Verification items for this drawing (mm, ordinates from the low corner). Round coordinates to 2 decimals unless told otherwise and drop trailing zeros. Order: outer loops, then holes, each group sorted by start corner. A loop starts at its lowest first (then second) coordinate and runs counter-clockwise, first axis right, second up. Notation, with made-up numbers: M 3,22 L 21,22 A6 cw 21,30 Z; hole C 21,68 d6. An arc over 180 degrees is marked long. Use CSV: the item, a comma, the result in double quotes. Start each with the question number.
Q1. Sectioned sample at A-A (z = 11.75). Enter the section's corners in (x, y), and give its area (3 significant figures).
Q2. Gauge pin test, flat ends, axial feed: pin 1 Ø2 at (y, z) = (49, 12.5) entering from -X; pin 2 Ø1.2 at (x, z) = (91.5, 12) entering from -Y; pin 3 Ø2 at (y, z) = (42.5, 12.5) entering from +X. Record the tip position at first contact, or that the pin passes through.
Q3. Sectioned sample at B-B (y = 52.5). Enter the section's corners in (x, z), and give its area (3 significant figures).
Q4. Mould release check, pull along Y, two halves, no side actions. Record for the marked faces 1 and 2: +Y half, -Y half, draft (parallel to the pull), parting line (faces both ways), or undercut.
Q5. Scan lines: line 1 (X direction, y = 70, z = 12.5); line 2 (Y direction, x = 36, z = 12.75); line 3 (Z direction, x = 92, y = 71). Record each from-to range of solid material in increasing order.
Q6. Sectioned sample at C-C (x = 27). Enter the section's corners in (y, z), and give its area (3 significant figures).
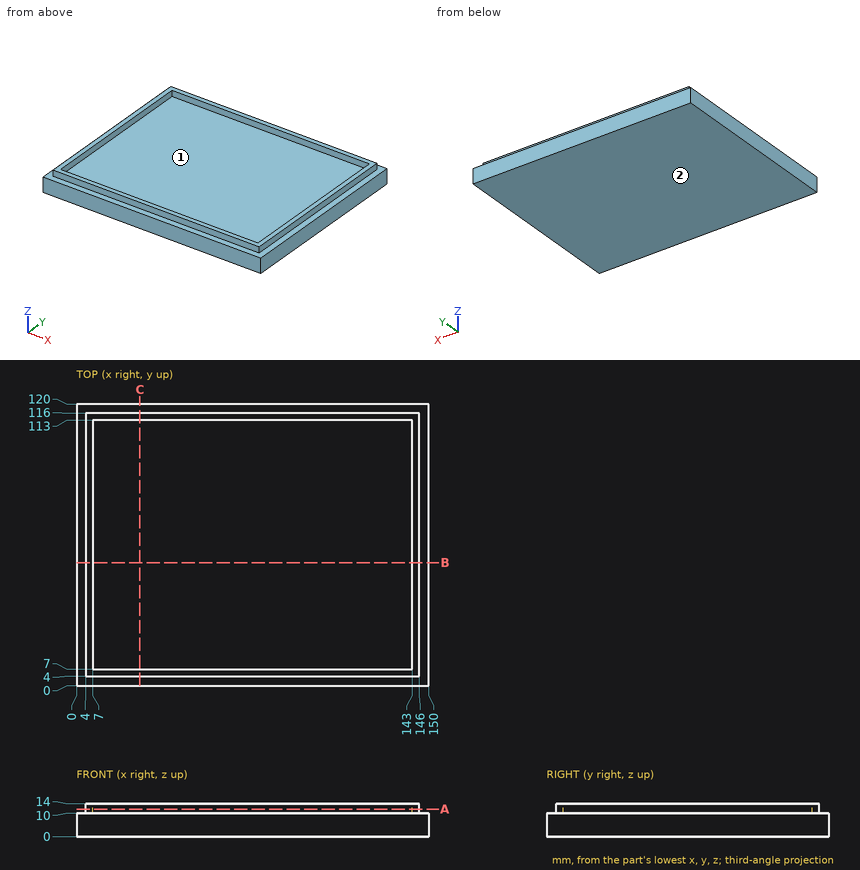
Verdict:
1,outline,"M 4,4 L 146,4 L 146,116 L 4,116 Z; hole M 7,7 L 143,7 L 143,113 L 7,113 Z"
1,area,"1,490 mm²"
2,pin 1,"stops at x = 4"
2,pin 2,"stops at y = 4"
2,pin 3,"stops at x = 146"
3,outline,"M 0,0 L 150,0 L 150,10 L 146,10 L 146,14 L 143,14 L 143,10 L 7,10 L 7,14 L 4,14 L 4,10 L 0,10 Z"
3,area,"1,520 mm²"
4,face 1,"undercut"
4,face 2,"draft"
5,line 1,"x = 4 to 7, 143 to 146"
5,line 2,"y = 4 to 7, 113 to 116"
5,line 3,"z = 0 to 10"
6,outline,"M 0,0 L 120,0 L 120,10 L 116,10 L 116,14 L 113,14 L 113,10 L 7,10 L 7,14 L 4,14 L 4,10 L 0,10 Z"
6,area,"1,220 mm²"
